Design review of the part shown in the three views and the two pictorial views. Dimensions are in mm from the part's minimum x, y and z. A direction names the side the tool comes from. Coordinates: 2 decimals unless noted, no trailing zeros. Loops run counter-clockwise (first coordinate to the right, second up) from the corner with the lowest first, then second, coordinate; pieces in that order, holes last. Notation, with made-up numbers: (-34.5, 41.5) -> (6.5, 41.5) arc R20 ccw to (6.5, 74.5) -> close; hole circle Ø11 at (64, 14.25). An arc over 180 degrees is marked (long way). Use CSV: the item, a comma, the result in double quotes.
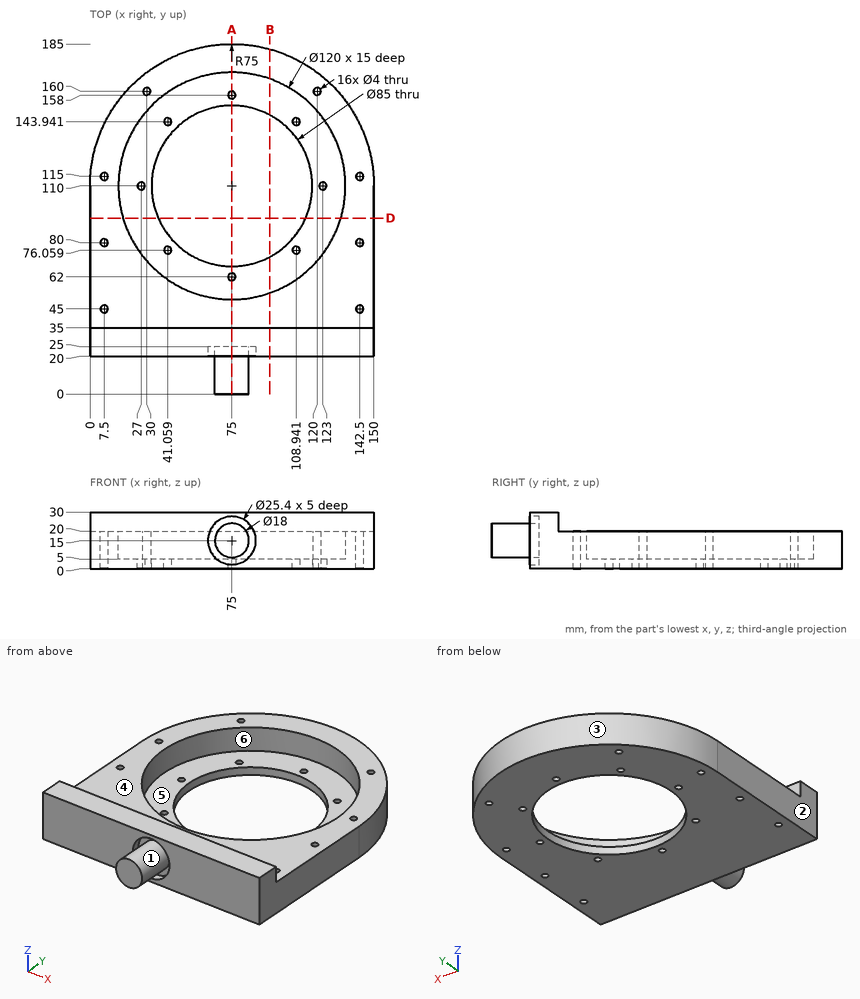
Item 1: Draft analysis for pull direction Y (two halves, no side actions). For the marked faces 3, 4, 5 and 6, state which applies: pulls with the +Y half, pulls with the -Y half, needs draft (parallel to the pull), parting line crosses it, or undercut.
Checked values:
face 3,"pulls with the +Y half"
face 4,"needs draft"
face 5,"undercut"
face 6,"undercut"
Item 2: Machinability: for the marked faces 1 and 2, which of the approach directions +Z, -Z, +X, -X, +Y, -Y give a long, thin tool a straight path to every point of the face, cutting with its end or side? Answer none if there is none.
Checked values:
face 1,"-Y"
face 2,"+Z, -Z, -X, +Y, -Y"
Item 3: Add section A-A (x = 75). State how many separate pieces and enclosed holes the cut face has, then the cut area to 3 significant figures.
Checked values:
separate pieces,"4"
enclosed holes,"0"
area,"1,510 mm^2"
Item 4: Clearance check with flat-ended pins moving along their axes: pin 1 (3.5 mm diameter, centred on x = 108.94, y = 143.94, fed in from +Z); pin 2 (2 mm diameter, centred on x = 130.5, z = 14.5, fed in from -Y); pin 3 (5 mm diameter, centred on x = 41.06, y = 143.94, fed in from +Z); pin 4 (1 mm diameter, centred on y = 157.5, z = 4, fed in from -X). State where each tip first meets the part, or that it passes through.
Checked values:
pin 1,"through"
pin 2,"y = 20"
pin 3,"z = 5"
pin 4,"x = 16.55"
Item 5: To check wall thickness, follow line 1 along Y through (x, z) = (142.5, 4); line 2 along Z through (x, y) = (32.5, 51.5); line 3 along Y through (x, z) = (120, 6.5). State the ranges of each line that lie inside material, in increasing order.
Checked values:
line 1,"20 to 43, 47 to 78, 82 to 113, 117 to 142.69"
line 2,"0 to 20"
line 3,"20 to 70.31, 149.69 to 158, 162 to 170"
Item 6: Add section B-B (x = 95). Give the boundary of the cut face in (y, z), then the cut area to 3 significant figures.
Checked values:
outline,"(20, 0) -> (72.5, 0) -> (72.5, 5) -> (53.43, 5) -> (53.43, 20) -> (35, 20) -> (35, 30) -> (20, 30) -> close; (147.5, 0) -> (182.28, 0) -> (182.28, 20) -> (166.57, 20) -> (166.57, 5) -> (147.5, 5) -> close"
area,"1,320 mm^2"
Item 7: Add section D-D (y = 93). Give the boundary of the cut face in (x, z), then the cut area to 3 significant figures.
Checked values:
outline,"(0, 0) -> (36.05, 0) -> (36.05, 5) -> (17.46, 5) -> (17.46, 20) -> (0, 20) -> close; (113.95, 0) -> (150, 0) -> (150, 20) -> (132.54, 20) -> (132.54, 5) -> (113.95, 5) -> close"
area,"884 mm^2"
